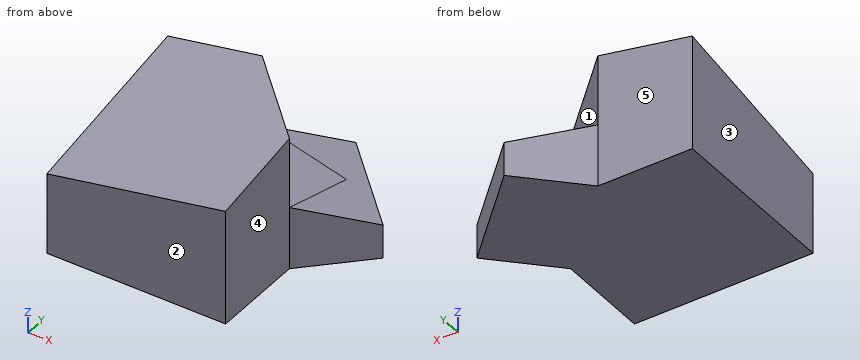
from build123d import *

# Parameters (mm, degrees)
F0_W     = 19.05
F0_H     = 19.05
F1_DEPTH = 15.875
F4_DEPTH = 18.796
F6_DEPTH = 6.35
F8_DEPTH = 12.7


with BuildPart() as f1:
    # F0 (on Top) → F1 (new body)
    with BuildSketch(Plane.XY):
        Rectangle(F0_W, F0_H)
    extrude(amount=F1_DEPTH)

    # F3 (on face) → F4 (cut, symmetric)
    with BuildSketch(Plane(origin=(0, 0, 0), x_dir=(0.707107, 0.707107, 0), z_dir=(0.707107, -0.707107, 0))):
        Polygon((-20.731339, 6.710676), (13.470384, 15.875), (-26.841145, 15.875), align=None)
    extrude(amount=F4_DEPTH, both=True, mode=Mode.SUBTRACT)

    # F5 (on face) → F6 (join, symmetric)
    with BuildSketch(Plane(origin=(0, 0, 0), x_dir=(0.707107, 0.707107, 0), z_dir=(0.707107, -0.707107, 0))):
        Polygon((5.318243, 0), (13.470384, 0), (25.414204, 0), (5.383082, 7.290732), align=None)
    extrude(amount=F6_DEPTH, both=True)

    # F7 (on face) → F8 (cut, symmetric)
    with BuildSketch(Plane(origin=(0, 0, 0), x_dir=(0.707107, 0.707107, 0), z_dir=(0.707107, -0.707107, 0))):
        Polygon((7.120384, 16.243063), (7.120384, 6.658406), (15.546197, 3.591661), (15.546197, 0), (25.414204, 0), (14.018306, 17.516766), align=None)
    extrude(amount=F8_DEPTH, both=True, mode=Mode.SUBTRACT)


solid = f1.part
CAD build for the part. Positions are in the model's coordinates, mm. Face numbers are marked on the shaded views. A direction names the side the tool comes from. Round coordinates to 2 decimals unless told otherwise and drop trailing zeros. Write each loop counter-clockwise with the first axis right and the second up, starting at its lowest first coordinate (ties: lowest second). Pieces come first, ordered by that corner, then holes.
(1) Slice it at B-B, the plane x = 3.5. Write the cut outline in (y, z) (3 decimals).
(2) Slice it at C-C, the plane y = 10.5. Write the cut outline in (x, z), and give its area (3 significant figures).
(3) Probe line 1 along X through (y, z) = (-0.75, 7.5) (3 decimals); line 2 along Z through (x, y) = (-1.25, -2.25). List the from-to ranges inside material, lowest first.
(4) 3-axis set-ups, long thin cutter, end or side, ignore diameter. For the marked faces 1, 2, 3, 4 and 5: which of +Z, -Z, +X, -X, +Y, -Y reach the whole face in a straight line?
(5) Slice it at D-D, the plane z = 10.25. Write the cut outline in (x, y) (3 decimals), and give its area (3 significant figures).
(6) Slice it at A-A, the plane z = 3.25. Write the cut outline in (x, y) (3 decimals).
(7) Drop flat-ended pins along their axis: P1, Ø8, axis at x = -3, z = 4.5, coming from the +Y side; P2, Ø10, axis at x = -2, y = -2, coming from the +Z side; P3, Ø1.5, axis at y = 10.5, z = 6.5, coming from the -X side. Give the stop position or say it passes through.
From the geometry:
1. outline: (-9.525, 0) - (12.48, 0) - (12.48, 5.137) - (6.57, 6.658) - (6.57, 14.174) - (-9.525, 11.124) - close
2. outline: (1.52, 0) - (11.49, 0) - (11.49, 3.59) - (1.52, 6.16) - close
2. area: 48.6 mm2
3. line 1: x = -9.525 to 9.525
3. line 2: z = 0 to 11.6
4. face 1: +Z, +X, +Y
4. face 2: +Z, -Z, +X, -X, -Y
4. face 3: +Z, -Z, -X, +Y, -Y
4. face 4: +Z, -Z, +X, -Y
4. face 5: +Z, -Z, -X, +Y
5. outline: (-9.525, -1.113) - (-1.113, -9.525) - (9.525, -9.525) - (9.525, 0.545) - (0.545, 9.525) - (-9.525, 9.525) - close
5. area: 287 mm2
6. outline: (-9.525, -9.525) - (9.525, -9.525) - (9.525, 0.545) - (15.483, 6.503) - (6.503, 15.483) - (0.545, 9.525) - (-9.525, 9.525) - close
7. P1: stops at y = 9.98
7. P2: stops at z = 12.85
7. P3: stops at x = 0.77
